Autodesk Inventor part; units mm, degrees
ref_plane "YZ Plane" through (0, 0, 0) normal (1, 0, 0) x (0, 1, 0)
ref_plane "XZ Plane" through (0, 0, 0) normal (0, 1, 0) x (-1, 0, 0)
ref_plane "XY Plane" through (0, 0, 0) normal (0, 0, 1) x (1, 0, 0)
sketch "Sketch1" plane through (0, 0, 0) normal (1, 0, 0) x (0, 1, 0)
  arc A0 (-1.9, 11.5447) -> (-11.7, 0) centre (0, 0) ccw
  line L0 (1.9, 11.5447) -> (1.9, 7.75)
  line L1 (1.9, 7.75) -> (-1.9, 7.75)
  line L2 (-1.9, 7.75) -> (-1.9, 11.5447)
  line L3 (0, 7.75) -> (0, 0) construction
  arc A1 (1.9, 11.5447) -> (-1.9, 11.5447) centre (0, 0) ccw construction
  circle A2 centre (0, 0) radius 3.75
  line L4 (11.7, 0) -> (11.7, -20)
  line L5 (11.7, -20) -> (-11.7, -20)
  line L6 (-11.7, -20) -> (-11.7, 0)
  arc A3 (11.7, 0) -> (1.9, 11.5447) centre (0, 0) ccw
  arc A4 (-11.7, 0) -> (11.7, 0) centre (0, 0) ccw construction
  dimension "d0" = 23.4
  dimension "d1" = 3.8
  dimension "d2" = 7.75
  dimension "d3" = 7.5
  dimension "d9" = 20
extrude "Extrusion1" add sketch "Sketch1" along normal blind 3
pattern_linear "Rectangular Pattern1" count 2 spacing 52.25 along (-1, 0, 0) of "Extrusion1"
sketch "Sketch3" plane through (0, -11.7, -20) normal (0, -1, 0) x (1, 0, 0)
  line L0 (-52.25, 0) -> (-49.25, 0)
  line L1 (-52.25, 0) -> (3, 0)
  line L2 (3, 0) -> (3, 23.5)
  line L3 (3, 23.5) -> (-52.25, 23.5)
  line L4 (-52.25, 23.5) -> (-52.25, 0)
  point P0 (0, 20)
  dimension "d12" = 3.5
extrude "Extrusion3" add sketch "Sketch3" along normal blind 3
sketch "Sketch4" plane through (0, -11.7, -20) normal (0, 1, 0) x (1, 0, 0)
  line L0 (-49.25, -31.5447) -> (-49.25, -20) construction
  line L1 (-49.25, -20) -> (-52.25, -20)
  line L2 (-52.25, -20) -> (-52.25, -23.5)
  line L3 (-52.25, -23.5) -> (-49.25, -23.5)
  line L4 (-49.25, -23.5) -> (-49.25, -20)
  line L5 (0, -20) -> (0, 0) construction
  line L6 (3, -23.5) -> (-52.25, -23.5) construction
  line L7 (0, -20) -> (3, -20)
  line L8 (3, -20) -> (3, -23.5)
  line L9 (3, -23.5) -> (0, -23.5)
  line L10 (0, -23.5) -> (0, -20)
extrude "Extrusion4" add sketch "Sketch4" along normal up to surface
mirror "Mirror1" about plane through (0, 0, 0) normal (0, 1, 0) of "Extrusion3", "Extrusion4"
sketch "Sketch9" plane through (-52.25, 14.7, -20) normal (0, 1, 0) x (1, 0, 0)
  circle A0 centre (12.625, -10) radius 2.8813
  circle A1 centre (42.625, -10) radius 2.8813
  line L0 (12.625, -10) -> (42.625, -10) construction
  line L1 (27.625, -10) -> (27.625, 0) construction
  line L2 (3, 0) -> (52.25, 0) construction
  point P0 (52.25, -20)
  dimension "d30" = 5.7625
  dimension "d31" = 30
  dimension "d32" = 10
extrude "Extrusion9" cut sketch "Sketch9" against normal up to surface (3 mm away)
sketch "Sketch10" plane through (0, -14.7, -20) normal (0, -1, 0) x (1, 0, 0)
  circle A0 centre (-9.625, 10) radius 5
  circle A1 centre (-39.625, 10) radius 5
  circle A2 centre (-39.625, 10) radius 2.8813 construction
  circle A3 centre (-9.625, 10) radius 2.8813 construction
  point P0 (0, 20)
  dimension "d35" = 10
extrude "Extrusion10" cut sketch "Sketch10" against normal up to surface (3 mm away)
properties part number "Xgantry_CableChain_bottom_connector"
Design review of the part built by this model. Coordinates are the model's own, in mm. A direction names the side the tool comes from. Coordinates: 2 decimals unless noted, no trailing zeros. Loops run counter-clockwise (first coordinate to the right, second up) from the corner with the lowest first, then second, coordinate; pieces in that order, holes last. Notation, with made-up numbers: M -20.5,65 L 3.5,65 A17 cw 3.5,76 Z; hole C 83,61.5 d6. An arc over 180 degrees is marked long. Answer as CSV lines item,"result".
Item 1: Add section D-D on x = -20. State the section outline as (y, z) points, plus the area to 3 significant figures.
Answer list:
outline,"M -14.7,-20 L -11.7,-20 L -11.7,3.5 L -14.7,3.5 Z; M 11.7,-20 L 14.7,-20 L 14.7,3.5 L 11.7,3.5 Z"
area,"141 mm²"
Item 2: The part is to be moulded in two halves that separate along Z. For faces 6 (the face through (-40.25, 13.221, -7.187)), 7 (the face through (-20, 12, -20)), 8 (the face through (-52.25, 0, -8)), say which applies: pulls with the +Z half, pulls with the -Z half, needs draft (parallel to the pull), parting line crosses it, or undercut.
Answer list:
face 6,"undercut"
face 7,"pulls with the -Z half"
face 8,"needs draft"
Item 3: Machinability: for faces 1 (the face through (-24, 14.7, -8)), 2 (the face through (-4.856, -13.221, -8.498)), 3 (the face through (-49.25, 0, -4)), 4 (the face through (-51, 1.9, 10)), 5 (the face through (-24, -13, 3.5)), which of the approach directions +Z, -Z, +X, -X, +Y, -Y give a long, thin tool a straight path to every point of the face, cutting with its end or side? Answer none if there is none.
Answer list:
face 1,"+Z, -Z, +X, -X, +Y"
face 2,"-Y"
face 3,"+Z, -Z"
face 4,"+Z, +X, -X"
face 5,"+Z, +X, -X, -Y"
Item 4: Add section A-A on z = 4.5. State the section outline as (x, y) points.
Answer list:
outline,"M -52.25,-10.8 L -49.25,-10.8 L -49.25,10.8 L -52.25,10.8 Z; M 0,-10.8 L 3,-10.8 L 3,10.8 L 0,10.8 Z"
Item 5: For P1, Ø2, axis at x = -13.5, y = -11, coming from the +Z side; P2, Ø0.9, axis at x = 1, z = 10.5, coming from the +Y side; P3, Ø2.5, axis at x = -50.5, y = 0.5, coming from the +Z side, all flat-tipped, find the tip position at first contact; note any pin that passes through.
Answer list:
P1,"z = 3.5"
P2,"y = 5.99"
P3,"z = 7.75"
Item 6: Add section B-B on y = 0. State the section outline as (x, z) points.
Answer list:
outline,"M -52.25,-20 L -49.25,-20 L -49.25,-3.75 L -52.25,-3.75 Z; M -52.25,3.75 L -49.25,3.75 L -49.25,7.75 L -52.25,7.75 Z; M 0,-20 L 3,-20 L 3,-3.75 L 0,-3.75 Z; M 0,3.75 L 3,3.75 L 3,7.75 L 0,7.75 Z"
Item 7: Add section C-C on z = -10. State the section outline as (x, y) points (3 decimals), plus the area to 3 significant figures.
Answer list:
outline,"M -52.25,-14.7 L -44.625,-14.7 L -44.625,-11.7 L -49.25,-11.7 L -49.25,11.7 L -42.506,11.7 L -42.506,14.7 L -52.25,14.7 Z; M -36.744,11.7 L -12.506,11.7 L -12.506,14.7 L -36.744,14.7 Z; M -34.625,-14.7 L -14.625,-14.7 L -14.625,-11.7 L -34.625,-11.7 Z; M -6.744,11.7 L 0,11.7 L 0,-11.7 L -4.625,-11.7 L -4.625,-14.7 L 3,-14.7 L 3,14.7 L -6.744,14.7 Z"
area,"377 mm²"
Item 8: For probe 1 along X at (y, z) = (13.2, -10); probe 2 along Y at (x, z) = (-4.5, -12.5); probe 3 along Z at (x, y) = (2.1, 0), list the stretches that pass through material, from the lowest coordinate up.
Answer list:
probe 1,"-52.25 to -42.51, -36.74 to -12.51, -6.74 to 3"
probe 2,"-14.7 to -11.7, 11.7 to 14.7"
probe 3,"-20 to -3.75, 3.75 to 7.75"
